The model under review builds one solid part; all positions refer to its coordinate system, in mm. A direction names the side the tool comes from. Coordinates: 2 decimals unless noted, no trailing zeros. Order: outer loops, then holes, each group sorted by start corner. A loop starts at its lowest first (then second) coordinate and runs counter-clockwise, first axis right, second up. Notation, with made-up numbers: (18.5, -5) -> (47.5, -5) arc R30 cw to (47.5, 20) -> close; hole circle Ø7 at (10.25, 1.25). An arc over 180 degrees is marked (long way). Answer as CSV lines item,"result". Start each with the question number.
from build123d import *

# Parameters (mm, degrees)
CROQUIS2_R              = 12.7
SALIENTE_EXTRUIR1_DEPTH = 12.7
CROQUIS4_R              = 12.7
SALIENTE_EXTRUIR4_DEPTH = 50.8
CORTAR_EXTRUIR1_START   = -12.7
CROQUIS4_5_R            = 12.7
CORTAR_EXTRUIR1_DEPTH   = 25.4


with BuildPart() as part:
    # Croquis2 → Saliente-Extruir1 (new body)
    with BuildSketch(Plane(origin=(0, 0, 0), x_dir=(1, 0, 0), z_dir=(0, 1, 0))):
        with BuildLine():
            Line((0, 0), (0, 50.8))
            Line((0, 50.8), (-88.9, 50.8))
            ThreePointArc((-88.9, 50.8), (-114.3, 25.4), (-88.9, 0))
            Line((-88.9, 0), (0, 0))
        make_face()
        with Locations(Location((-88.9, 25.4, 0), (0, 0, 270))):
            Circle(CROQUIS2_R, mode=Mode.SUBTRACT)
    extrude(amount=SALIENTE_EXTRUIR1_DEPTH)

    # Croquis4 → Saliente-Extruir4 (add, through all)
    with BuildSketch(Plane.XY):
        with BuildLine():
            Line((0, 12.7), (0, 38.1))
            ThreePointArc((0, 38.1), (-25.4, 63.5), (-50.8, 38.1))
            Line((-50.8, 38.1), (-50.8, 12.7))
            Line((-50.8, 12.7), (0, 12.7))
        make_face()
        with Locations((-25.4, 38.1)):
            Circle(CROQUIS4_R, mode=Mode.SUBTRACT)
    extrude(amount=-SALIENTE_EXTRUIR4_DEPTH)

    # Croquis4<5> → Cortar-Extruir1 (cut)
    with BuildSketch(Plane.XY.offset(CORTAR_EXTRUIR1_START)):
        with BuildLine():
            Line((0, 12.7), (0, 38.1))
            ThreePointArc((0, 38.1), (-25.4, 63.5), (-50.8, 38.1))
            Line((-50.8, 38.1), (-50.8, 12.7))
            Line((-50.8, 12.7), (0, 12.7))
        make_face()
        with Locations((-25.4, 38.1)):
            Circle(CROQUIS4_5_R, mode=Mode.SUBTRACT)
    extrude(amount=-CORTAR_EXTRUIR1_DEPTH, mode=Mode.SUBTRACT)


solid = part.part
1) Consider section A-A (x = -25.4). Give the boundary of the cut face in (y, z).
2) Tool access review of faces 1 (the face through (-50.8, 26, -44)), 2 (the face through (-26, 22, -12.7)), 3 (the face through (-35, 25, 0)): name each direction out of +Z, -Z, +X, -X, +Y, -Y from which nothing blocks a thin tool from reaching the whole face with its end or side.
3) Consider section B-B (z = -25.4). Give the boundary of the cut face in (x, y).
4) Consider section C-C (y = 20). Give the boundary of the cut face in (x, z).
5) Insertion check: pin 1 Ø14 at (y, z) = (21.5, -47.5) entering from -X; pin 2 Ø2 at (y, z) = (46.5, -39.5) entering from +X; pin 3 Ø3 at (x, z) = (-35.5, -6) entering from +Y; pin 4 Ø20.5 at (x, z) = (-88.9, -25.4) entering from +Y. Each pin has a flat end and moves straight along its axis. Give the tip position at first contact, or say it passes through.
6) Mouldability with a two-part tool opening along Y and no side actions: class faces 4 (the face through (-18.573, 48.809, -6.261)), 5 (the face through (-58, 0, -26)), 6 (the face through (-114.294, 6.261, -25.959)), 7 (the face through (-24.841, 63.494, -6.261)) as released by +Y, released by -Y, zero draft, split by the parting line, or undercut.
7) Wall thickness on L1, parallel to X at y = 38, z = -5; L2, parallel to Y at x = -25, z = -42; L3, parallel to X at y = 8, z = -25: over which ranges is each line inside the solid? List them lowest first. Write a range as [from, to].
8) Consider section D-D (y = 47). Give the boundary of the cut face in (x, z), plus the area to 3 significant figures.
Result:
1,outline,"(0, -50.8) -> (25.4, -50.8) -> (25.4, -38.1) -> (12.7, -38.1) -> (12.7, -12.7) -> (25.4, -12.7) -> (25.4, 0) -> (0, 0) -> close; (50.8, -50.8) -> (63.5, -50.8) -> (63.5, -38.1) -> (50.8, -38.1) -> close; (50.8, -12.7) -> (63.5, -12.7) -> (63.5, 0) -> (50.8, 0) -> close"
2,face 1,"+Z, -Z, -X, +Y"
2,face 2,"+X, -X, +Y"
2,face 3,"+Z, +X, -X, +Y, -Y"
3,outline,"(-114.3, 0) -> (-101.6, 0) -> (-101.6, 12.7) -> (-114.3, 12.7) -> close; (-76.2, 0) -> (0, 0) -> (0, 12.7) -> (-76.2, 12.7) -> close"
4,outline,"(-50.8, -50.8) -> (0, -50.8) -> (0, -38.1) -> (-50.8, -38.1) -> close; (-50.8, -12.7) -> (0, -12.7) -> (0, 0) -> (-50.8, 0) -> close"
5,pin 1,"x = -50.8"
5,pin 2,"x = -1.1"
5,pin 3,"y = 62"
5,pin 4,"through"
6,face 4,"undercut"
6,face 5,"released by -Y"
6,face 6,"zero draft"
6,face 7,"released by +Y"
7,L1,"[-50.8, -38.1], [-12.7, 0]"
7,L2,"[0, 25.41], [50.79, 63.5]"
7,L3,"[-114.3, -101.59], [-76.21, 0]"
8,outline,"(-49.19, -50.8) -> (-34.46, -50.8) -> (-34.46, -38.1) -> (-49.19, -38.1) -> close; (-49.19, -12.7) -> (-34.46, -12.7) -> (-34.46, 0) -> (-49.19, 0) -> close; (-16.34, -50.8) -> (-1.61, -50.8) -> (-1.61, -38.1) -> (-16.34, -38.1) -> close; (-16.34, -12.7) -> (-1.61, -12.7) -> (-1.61, 0) -> (-16.34, 0) -> close"
8,area,"748 mm2"
